from build123d import *

# Parameters (mm, degrees)
BASE_FLANGE1_DEPTH             = 241.3
SKETCH7_W                      = 38.1
SKETCH7_H                      = 114.3
CUT_EXTRUDE2_DEPTH             = 25.4
EDGE_FLANGE1_DEPTH             = 63.5
FILLET2_R                      = 6.35
F_3_16_0_1875_DIAMETER_HOLE2_D = 4.7625
CUT_EXTRUDE1_REACH             = 293.504
CUT_EXTRUDE3_REACH             = 294.454
CUT_EXTRUDE4_REACH             = 294.454
SKETCH12_W                     = 317.5
SKETCH12_H                     = 25.4
FILLET1_R                      = 3.175
FILLET3_R                      = 9.525
CUT_EXTRUDE5_REACH             = 294.057


# Sheet-metal steps are written as plain solids
with BuildPart() as part:
    # Sketch1 → Base-Flange1 (new, symmetric)
    with BuildSketch(Plane.XY):
        with BuildLine():
            Line((0, 88.9), (0, 6.35))
            ThreePointArc((0, 6.35), (-1.859871939, 1.859871939), (-6.35, 0))
            Line((-6.35, 0), (-38.1, 0))
            Line((-38.1, 0), (-38.1, 3.175))
            Line((-38.1, 3.175), (-6.35, 3.175))
            ThreePointArc((-6.35, 3.175), (-4.10493597, 4.10493597), (-3.175, 6.35))
            Line((-3.175, 6.35), (-3.175, 88.9))
            Line((-3.175, 88.9), (0, 88.9))
        make_face()
    extrude(amount=BASE_FLANGE1_DEPTH, both=True)

    # Sketch7 → Cut-Extrude2 (cut)
    with BuildSketch(Plane.XZ):
        with Locations((-19.05, -184.15)):
            Rectangle(SKETCH7_W, SKETCH7_H)
    extrude(amount=-CUT_EXTRUDE2_DEPTH, mode=Mode.SUBTRACT)

    # Edge-Flange1 section (across the edge) → Edge-Flange1 (add)
    with BuildSketch(Plane(origin=(-3.175, 88.9, -242.150738686), x_dir=(-0.8660254037844416, 0, 0.49999999999999495), z_dir=(0, -1, 0))):
        with BuildLine():
            Line((-3.175, 0.850738686), (-3.175, 37.249261314))
            Line((-3.175, 37.249261314), (0, 37.249261314))
            Line((0, 37.249261314), (0, 0.850738686))
            ThreePointArc((0, 0.850738686), (0.108185502, 0.028988218), (0.425369343, -0.736761314))
            Line((0.425369343, -0.736761314), (-2.324261314, -2.324261314))
            ThreePointArc((-2.324261314, -2.324261314), (-2.958628997, -0.79276225), (-3.175, 0.850738686))
        make_face()
    extrude(amount=EDGE_FLANGE1_DEPTH)

    # Fillet2
    fillet2_edges = [part.edges().sort_by_distance(p)[0] for p in [
        (-20.424815329, 88.9, -275.203295256),
        (-20.424815329, 25.4, -275.203295256),
    ]]
    fillet(fillet2_edges, radius=FILLET2_R)

    # 3/16 (0.1875) Diameter Hole2 (through all)
    with Locations(Plane(origin=(0, 0, 0), x_dir=(0, 0, -1), z_dir=(1, 0, 0))):
        with Locations((111.91875, 36.5125), (162.71875, 36.5125)):
            Hole(F_3_16_0_1875_DIAMETER_HOLE2_D / 2)

    # Sketch5 → Cut-Extrude1 (cut, up to next)
    with BuildSketch(Plane(origin=(0, 3.175, 0), x_dir=(-1, 0, 0), z_dir=(0, 1, 0)), mode=Mode.PRIVATE) as cut_extrude1_sk1:
        with BuildLine():
            Line((28.575, -117.871875), (15.875, -117.871875))
            ThreePointArc((15.875, -117.871875), (12.303125, -114.3), (15.875, -110.728125))
            Line((15.875, -110.728125), (28.575, -110.728125))
            ThreePointArc((28.575, -110.728125), (32.146875, -114.3), (28.575, -117.871875))
        make_face()
    cut_extrude1_tool1 = extrude(cut_extrude1_sk1.sketch, amount=-CUT_EXTRUDE1_REACH, mode=Mode.PRIVATE) & part.part
    # Sketch5 → Cut-Extrude1 (cut, up to next)
    with BuildSketch(Plane(origin=(0, 3.175, 0), x_dir=(-1, 0, 0), z_dir=(0, 1, 0)), mode=Mode.PRIVATE) as cut_extrude1_sk2:
        with BuildLine():
            Line((28.575, 225.028125), (15.875, 225.028125))
            ThreePointArc((15.875, 225.028125), (12.303125, 228.6), (15.875, 232.171875))
            Line((15.875, 232.171875), (28.575, 232.171875))
            ThreePointArc((28.575, 232.171875), (32.146875, 228.6), (28.575, 225.028125))
        make_face()
    cut_extrude1_tool2 = extrude(cut_extrude1_sk2.sketch, amount=-CUT_EXTRUDE1_REACH, mode=Mode.PRIVATE) & part.part
    add(cut_extrude1_tool1.solids().sort_by_distance((-22.225, 3.175, -114.3))[0], mode=Mode.SUBTRACT)
    add(cut_extrude1_tool2.solids().sort_by_distance((-22.225, 3.175, 228.6))[0], mode=Mode.SUBTRACT)

    # Sketch11 → Cut-Extrude3 (cut, up to next)
    with BuildSketch(Plane(origin=(0, 0, 0), x_dir=(0, 0, -1), z_dir=(1, 0, 0)), mode=Mode.PRIVATE) as cut_extrude3_sk1:
        with BuildLine():
            Line((115.09375, 41.275), (115.09375, 31.75))
            ThreePointArc((115.09375, 31.75), (111.91875, 28.575), (108.74375, 31.75))
            Line((108.74375, 31.75), (108.74375, 41.275))
            ThreePointArc((108.74375, 41.275), (111.91875, 44.45), (115.09375, 41.275))
        make_face()
    cut_extrude3_tool1 = extrude(cut_extrude3_sk1.sketch, amount=-CUT_EXTRUDE3_REACH, mode=Mode.PRIVATE) & part.part
    # Sketch11 → Cut-Extrude3 (cut, up to next)
    with BuildSketch(Plane(origin=(0, 0, 0), x_dir=(0, 0, -1), z_dir=(1, 0, 0)), mode=Mode.PRIVATE) as cut_extrude3_sk2:
        with BuildLine():
            Line((165.89375, 41.275), (165.89375, 31.75))
            ThreePointArc((165.89375, 31.75), (162.71875, 28.575), (159.54375, 31.75))
            Line((159.54375, 31.75), (159.54375, 41.275))
            ThreePointArc((159.54375, 41.275), (162.71875, 44.45), (165.89375, 41.275))
        make_face()
    cut_extrude3_tool2 = extrude(cut_extrude3_sk2.sketch, amount=-CUT_EXTRUDE3_REACH, mode=Mode.PRIVATE) & part.part
    add(cut_extrude3_tool1.solids().sort_by_distance((0, 36.5125, -111.91875))[0], mode=Mode.SUBTRACT)
    add(cut_extrude3_tool2.solids().sort_by_distance((0, 36.5125, -162.71875))[0], mode=Mode.SUBTRACT)

    # Sketch12 → Cut-Extrude4 (cut, up to next)
    with BuildSketch(Plane(origin=(0, 0, 0), x_dir=(0, 0, -1), z_dir=(1, 0, 0)), mode=Mode.PRIVATE) as cut_extrude4_sk1:
        with Locations((-57.15, 12.7)):
            Rectangle(SKETCH12_W, SKETCH12_H)
    cut_extrude4_tool1 = extrude(cut_extrude4_sk1.sketch, amount=-CUT_EXTRUDE4_REACH, mode=Mode.PRIVATE) & part.part
    add(cut_extrude4_tool1.solids().sort_by_distance((0, 12.7, 57.15))[0], mode=Mode.SUBTRACT)

    # Fillet1
    fillet1_edges = [part.edges().sort_by_distance(p)[0] for p in [
        (-38.1, 1.5875, 215.9),
        (-38.1, 1.5875, -101.6),
        (-1.5875, 88.9, 241.3),
        (-38.1, 1.5875, -127),
        (-38.1, 1.5875, 241.3),
    ]]
    fillet(fillet1_edges, radius=FILLET1_R)

    # Fillet3
    fillet3_edges = [part.edges().sort_by_distance(p)[0] for p in [
        (-1.5875, 25.4, 215.9),
        (-1.5875, 25.4, -101.6),
        (-1.5875, 25.4, -127),
    ]]
    fillet(fillet3_edges, radius=FILLET3_R)

    # Sketch13 → Cut-Extrude5 (cut, up to next)
    with BuildSketch(Plane.ZY.offset(3.175), mode=Mode.PRIVATE) as cut_extrude5_sk1:
        with BuildLine():
            Line((-19.64055, 74.6125), (-19.64055, 61.9125))
            ThreePointArc((-19.64055, 61.9125), (-23.01875, 58.5343), (-26.39695, 61.9125))
            Line((-26.39695, 61.9125), (-26.39695, 74.6125))
            ThreePointArc((-26.39695, 74.6125), (-23.01875, 77.9907), (-19.64055, 74.6125))
        make_face()
    cut_extrude5_tool1 = extrude(cut_extrude5_sk1.sketch, amount=-CUT_EXTRUDE5_REACH, mode=Mode.PRIVATE) & part.part
    # Sketch13 → Cut-Extrude5 (cut, up to next)
    with BuildSketch(Plane.ZY.offset(3.175), mode=Mode.PRIVATE) as cut_extrude5_sk2:
        with BuildLine():
            Line((101.00945, 74.6125), (101.00945, 61.9125))
            ThreePointArc((101.00945, 61.9125), (97.63125, 58.5343), (94.25305, 61.9125))
            Line((94.25305, 61.9125), (94.25305, 74.6125))
            ThreePointArc((94.25305, 74.6125), (97.63125, 77.9907), (101.00945, 74.6125))
        make_face()
    cut_extrude5_tool2 = extrude(cut_extrude5_sk2.sketch, amount=-CUT_EXTRUDE5_REACH, mode=Mode.PRIVATE) & part.part
    add(cut_extrude5_tool1.solids().sort_by_distance((-3.175, 68.2625, -23.01875))[0], mode=Mode.SUBTRACT)
    add(cut_extrude5_tool2.solids().sort_by_distance((-3.175, 68.2625, 97.63125))[0], mode=Mode.SUBTRACT)


solid = part.part
Here's how the part is built. I have some questions about the finished solid (model axes, mm). A direction names the side the tool comes from. Coordinates: 2 decimals unless noted, no trailing zeros. Loops run counter-clockwise (first coordinate to the right, second up) from the corner with the lowest first, then second, coordinate; pieces in that order, holes last.
1. If we mould it in two halves opening along Z, with no side actions, what happens to faces 6 (the flat face through (-12, 3, -101.6)), 7 (the flat face through (-14, 3, -127)), 8 (the flat face through (-3, 37, 241.3))? For each: pulls with the +Z half, pulls with the -Z half, needs draft (parallel to the pull), parting line crosses it, or undercut.
2. For P1, Ø5, axis at x = -13, y = 42, coming from the -Z side; P2, Ø2.5, axis at x = -1.5, y = 38, coming from the -Z side; P3, Ø3.5, axis at x = -24.5, y = 2, coming from the -Z side, each with a flat end and sliding along its axis, tell me the tip position at first contact or that it passes through.
3. For faces 1 (the flat face through (-9.823, 57.594, -260.015)), 2 (the flat face through (-1, 25.4, -197)), 3 (the flat face through (-22, 3.175, -120)), 4 (the flat face through (-3.175, 56, 3)), 5 (the flat face through (-12, 3, 215.9)), which set-ups out of +Z, -Z, +X, -X, +Y, -Y let a thin tool reach every point of the face, with its end or its side?
4. I need wall thicknesses on L1, parallel to Z at x = -2, y = 14.5; L2, parallel to X at y = 45, z = 215 (3 decimals); L3, parallel to Z at x = -17.5, y = 58.5. Which ranges of each line are inside material? Lowest first, please.
5. Imagine slicing it at A-A, the plane z = 196. Please give me the cut outline in (x, y) (3 decimals).
Taken from the geometry:
1. face 6: undercut
1. face 7: pulls with the -Z half
1. face 8: pulls with the +Z half
2. P1: stops at z = -269.85
2. P2: stops at z = -247.76
2. P3: stops at z = -127
3. face 1: -Z, +X, +Y, -Y
3. face 2: -Z, +X, -X, -Y
3. face 3: +Z, -Z, -X, +Y
3. face 4: +Z, -X, +Y
3. face 5: +X, -X, -Y
4. L1: z = -127 to -101.6, 215.9 to 241.3
4. L2: x = -3.175 to 0
4. L3: z = -273.31 to -266.96
5. outline: (-3.175, 25.4) - (0, 25.4) - (0, 88.9) - (-3.175, 88.9) - close
